Autodesk Inventor part; units mm, degrees
ref_plane "YZ Plane" through (0, 0, 0) normal (1, 0, 0) x (0, 1, 0)
ref_plane "XZ Plane" through (0, 0, 0) normal (0, 1, 0) x (-1, 0, 0)
ref_plane "XY Plane" through (0, 0, 0) normal (0, 0, 1) x (1, 0, 0)
sketch "Эскиз1" plane through (0, 0, 0) normal (1, 0, 0) x (0, 1, 0)
  line L0 (0, 0) -> (10, 0)
  line L1 (10, 0) -> (10, 40)
  line L2 (10, 40) -> (0, 40)
  line L3 (0, 40) -> (0, 0)
  line L4 (10, 40) -> (-70, 40)
  line L5 (-70, 40) -> (-70, 30)
  line L6 (-70, 30) -> (10, 30)
  line L7 (10, 30) -> (10, 40)
  circle A0 centre (5, 5) radius 2
  line L8 (-70, 40) -> (-60, 40)
  line L9 (-60, 40) -> (-60, 12)
  line L10 (-60, 12) -> (-70, 12)
  line L11 (-70, 12) -> (-70, 40)
  circle A1 centre (-65, 17) radius 2
  point P0 (5, 0)
  point P1 (0, 40)
  point P2 (0, 30)
  point P3 (-70, 35)
  point P4 (-65, 12)
  point P5 (-60, 30)
  point P6 (-70, 30)
  dimension "d0" = 10
  dimension "d1" = 10
  dimension "d2" = 40
  dimension "d3" = 4
  dimension "d4" = 5
  dimension "d5" = 5
  dimension "d6" = 80
  dimension "d13" = 28
  dimension "d14" = 10
  dimension "d15" = 5
extrude "Выдавливание1" add sketch "Эскиз1" along normal blind 10
fillet "Сопряжение1" radius 5 7 edges at (5, 0, 30) (5, 10, 40) (5, 10, 0) (5, 0, 0) (5, -70, 40) (5, -60, 12) (5, -70, 12)
properties part number "колено для сервы"
Verification items for the finished model (mm, model axes). A direction names the side the tool comes from. Coordinates: 2 decimals unless noted, no trailing zeros. Loops run counter-clockwise (first coordinate to the right, second up) from the corner with the lowest first, then second, coordinate; pieces in that order, holes last. Notation, with made-up numbers: (-34, 5.5) -> (-19, 5.5) arc R18 cw to (-19, 24.5) -> close; hole circle Ø3 at (62, 14.5). An arc over 180 degrees is marked (long way). Put each result on its own line as item: value.
1. Tool access check on faces 1 (the face through (5, -60, 24)), 2 (the face through (5, 9, 38)). Record the directions out of +Z, -Z, +X, -X, +Y, -Y that give a thin tool (end or side, any length) a straight path to the whole face; none if there is none.
Result set:
face 1: -Z, +X, -X
face 2: +Z, +X, -X, +Y
2. Section check A-A, the plane x = 3. Give the number of separate pieces and of enclosed holes in the cut face, then the cut area to 3 significant figures.
Result set:
separate pieces: 1
enclosed holes: 2
area: 1,230 mm^2
3. Section check B-B, the plane z = 8. Record the boundary of the cut face in (x, y), then the cut area to 3 significant figures.
Result set:
outline: (0, 0) -> (10, 0) -> (10, 10) -> (0, 10) -> close
area: 100 mm^2
4. Section check C-C, the plane y = -1. Record the boundary of the cut face in (x, z).
Result set:
outline: (0, 28) -> (10, 28) -> (10, 40) -> (0, 40) -> close
5. Gauge pin test, flat ends, axial feed: P1, Ø3, axis at y = -8, z = 31, coming from the -X side; P2, Ø5, axis at x = 6.5, y = -31.5, coming from the -Z side. Record the tip position at first contact, or that the pin passes through.
Result set:
P1: stops at x = 0
P2: stops at z = 30
6. Mould release check, pull along Y, two halves, no side actions. Record for faces 3 (the face through (10, -27, 32)), 4 (the face through (4.9, 3.4, 6.2)), 5 (the face through (5, 8, 1)): pulls with the +Y half, pulls with the -Y half, needs draft (parallel to the pull), parting line crosses it, or undercut.
Result set:
face 3: needs draft
face 4: undercut
face 5: pulls with the +Y half
7. Thickness scan on line 1 (Z direction, x = 7.75, y = -65); line 2 (Z direction, x = 2.5, y = 5); line 3 (Y direction, x = 9.25, z = 24). Record the ranges inside material, lowest first.
Result set:
line 1: z = 12 to 15, 19 to 40
line 2: z = 0 to 3, 7 to 40
line 3: y = -70 to -60, 0 to 10
